from build123d import *

# Parameters (mm, degrees)
SKETCH2_R           = 23.335
SKETCH2_R_2         = 13.335
BOSS_EXTRUDE1_DEPTH = 6
SKETCH3_R           = 2.5
SKETCH4_R           = 1.625
CUT_EXTRUDE1_DEPTH  = 7


with BuildPart() as part:
    # Sketch2 → Boss-Extrude1 (new body)
    with BuildSketch(Plane.XY):
        Circle(SKETCH2_R)
        Circle(SKETCH2_R_2, mode=Mode.SUBTRACT)
    extrude(amount=BOSS_EXTRUDE1_DEPTH)

    # Sketch3 → Cut-Revolve1 (revolve, cut)
    with BuildSketch(Plane(origin=(0, 0, 0), x_dir=(1, 0, 0), z_dir=(0, 1, 0))):
        with Locations((-23.335, 0)):
            Circle(SKETCH3_R)
        with Locations((-23.335, -6)):
            Circle(SKETCH3_R)
    revolve(axis=Axis((0, 0, 6), (0, 0, -1)), mode=Mode.SUBTRACT)

    # Sketch4 → Cut-Extrude1 (cut, through all)
    with BuildSketch(Plane(origin=(0, 0, 0), x_dir=(-1, 0, 0), z_dir=(0, 0, -1))):
        with Locations((8.5425, 14.796044024)):
            Circle(SKETCH4_R)
        with Locations((-8.5425, 14.796044024)):
            Circle(SKETCH4_R)
        with Locations((-17.085, 0)):
            Circle(SKETCH4_R)
        with Locations((-8.5425, -14.796044024)):
            Circle(SKETCH4_R)
        with Locations((8.5425, -14.796044024)):
            Circle(SKETCH4_R)
        with Locations((17.085, 0)):
            Circle(SKETCH4_R)
    extrude(amount=-CUT_EXTRUDE1_DEPTH, mode=Mode.SUBTRACT)


solid = part.part
Part model, mm, in its own coordinate system. Coordinates: 2 decimals unless noted, no trailing zeros. Write each loop counter-clockwise with the first axis right and the second up, starting at its lowest first coordinate (ties: lowest second). Pieces come first, ordered by that corner, then holes. Notation, with made-up numbers: (87.5, -29.75) - (104.5, -29.75) arc R20 ccw to (104.5, 4.25) - close; hole circle Ø10 at (40.25, 83.25). An arc over 180 degrees is marked (long way). Put each result on its own line as item: value.
1. Band-saw the part on B-B (y = 0). Write the cut outline in (x, z) (3 decimals), then the cut area to 3 significant figures.
Final values:
outline: (-23.335, 2.5) arc R2.5 cw to (-20.835, 0) - (-18.71, 0) - (-18.71, 6) - (-20.835, 6) arc R2.5 cw to (-23.335, 3.5) - close; (-15.46, 0) - (-13.335, 0) - (-13.335, 6) - (-15.46, 6) - close; (13.335, 0) - (15.46, 0) - (15.46, 6) - (13.335, 6) - close; (18.71, 0) - (20.835, 0) arc R2.5 cw to (23.335, 2.5) - (23.335, 3.5) arc R2.5 cw to (20.835, 6) - (18.71, 6) - close
area: 61.4 mm²
2. Flat gauge pins, fed straight in: pin 1 Ø3.5 at (x, y) = (-8.54, -14.8) entering from +Z; pin 2 Ø6 at (x, y) = (0, 9) entering from +Z; pin 3 Ø1 at (y, z) = (-10.5, 1) entering from +X; pin 4 Ø2 at (x, z) = (-14.5, 1) entering from +Y. Where does each tip first touch, or does it go through?
Final values:
pin 1: stops at z = 6
pin 2: passes through
pin 3: stops at x = 18.66
pin 4: stops at y = 16.54
3. Two-plate mould, pull along Y, no slides. Class faces 1 (the cylindrical face through (-8.331, -13.185, 2.958)), 2 (the flat face through (0, -14, 6)), 3 (the cylindrical face through (-5.06, -22.78, 2.99)), 4 (the cylindrical face through (10.166, 14.867, 2.958)): +Y half, -Y half, draft (parallel to the pull), parting line (faces both ways), or undercut.
Final values:
face 1: undercut
face 2: draft
face 3: parting line
face 4: undercut
4. Band-saw the part on A-A (x = 0). Write the cut outline in (y, z) (3 decimals).
Final values:
outline: (-23.335, 2.5) arc R2.5 cw to (-20.835, 0) - (-13.335, 0) - (-13.335, 6) - (-20.835, 6) arc R2.5 cw to (-23.335, 3.5) - close; (13.335, 0) - (20.835, 0) arc R2.5 cw to (23.335, 2.5) - (23.335, 3.5) arc R2.5 cw to (20.835, 6) - (13.335, 6) - close
5. Band-saw the part on C-C (z = 1.55). Give the number of separate pieces and of enclosed holes in the cut face, then the cut area to 3 significant figures.
Final values:
separate pieces: 1
enclosed holes: 7
area: 827 mm²
6. Probe line 1 along Y through (x, z) = (9, 0.45); line 2 along X through (y, z) = (-15, 0.9); line 3 along X through (y, z) = (14, 1.25). List the from-to ranges inside material, lowest first. Write a range as [from, to].
Final values:
line 1: y = [-18.84, -16.36], [-13.24, -9.84], [9.84, 13.24], [16.36, 18.84]
line 2: x = [-14.7, -10.15], [-6.93, 6.93], [10.15, 14.7]
line 3: x = [-15.88, -9.96], [-7.13, 7.13], [9.96, 15.88]
